from build123d import *

# Parameters (mm, degrees)
SKETCH_1_W         = 25.5
SKETCH_1_H         = 25
EXTRUDE_1_DEPTH    = 4
SKETCH_6_W         = 25.5
SKETCH_6_H         = 7
EXTRUDE_2_DEPTH    = 7
HOLE_WIZARD_M3_1_D = 2.5
HOLE_WIZARD_M4_3_D = 3.3
FILLET_1_R         = 1


with BuildPart() as part:
    # 草图1 → 凸台-拉伸1 (new body)
    with BuildSketch(Plane(origin=(0, 0, 0), x_dir=(1, 0, 0), z_dir=(0, 1, 0))):
        Rectangle(SKETCH_1_W, SKETCH_1_H)
    extrude(amount=EXTRUDE_1_DEPTH)

    # 草图6 → 凸台-拉伸2 (add)
    with BuildSketch(Plane(origin=(0, 4, 0), x_dir=(1, 0, 0), z_dir=(0, 1, 0))):
        with Locations((0, 9)):
            Rectangle(SKETCH_6_W, SKETCH_6_H)
        with Locations((0, -9)):
            Rectangle(SKETCH_6_W, SKETCH_6_H)
    extrude(amount=EXTRUDE_2_DEPTH)

    # M3 螺纹孔1 (through all)
    with Locations(Plane(origin=(6.35, 0, 0), x_dir=(0, 0, -1), z_dir=(0, -1, 0))):
        with Locations((0, 0), (0, -12.7)):
            Hole(HOLE_WIZARD_M3_1_D / 2)

    # M4 螺纹孔3 (through all)
    with Locations(Plane(origin=(7.5, 0, 8.5), x_dir=(0, 0, -1), z_dir=(0, -1, 0))):
        with Locations((0, 0), (0, -15), (17, -15), (17, 0)):
            Hole(HOLE_WIZARD_M4_3_D / 2)

    # 圆角1
    fillet_1_edges = [part.edges().sort_by_distance(p)[0] for p in [
        (0, 4, -5.5),
        (0, 11, -12.5),
        (0, 4, 5.5),
        (0, 11, 12.5),
        (0, 0, 12.5),
        (0, 0, -12.5),
    ]]
    fillet(fillet_1_edges, radius=FILLET_1_R)


solid = part.part
Geometry: final body of the model. Coordinates: model frame, mm. A direction names the side the tool comes from. Coordinates: 2 decimals unless noted, no trailing zeros. Order: outer loops, then holes, each group sorted by start corner. A loop starts at its lowest first (then second) coordinate and runs counter-clockwise, first axis right, second up. Notation, with made-up numbers: M -38.75,70.5 L -10.75,70.5 A32 ccw -10.75,98.5 Z; hole C 75.25,-22 d11. An arc over 180 degrees is marked long. One line per question, with ' | ' between items. Start each with the question number.
Item 1: Ray query, probe 1 along X at (y, z) = (6.75, -8.5); probe 2 along X at (y, z) = (2.55, 0); probe 3 along Z at (x, y) = (-4.75, 7.5). Return the intervals inside material, ascending. Write a range as [from, to].
Item 2: Cut plane C-C, the plane y = 3.5. Return the cut outline in (x, z), then the cut area to 3 significant figures.
Item 3: Cut plane B-B, the plane z = 8.5. Return the cut outline in (x, y), then the cut area to 3 significant figures.
Item 4: Cut plane D-D, the plane x = 6.35. Return the cut outline in (y, z).
Item 5: Draft query along Z for faces 1 (the cylindrical face through (0.178, 10.699, 12.215)), 2 (the flat face through (0, 11, 8)), 3 (the cylindrical face through (8.615, 5.577, 7.284)). Return one class per face: released by +Z, released by -Z, zero draft, split by the parting line, or undercut.
Item 6: Set-up query: faces 4 (the flat face through (12.75, 3, 0)), 5 (the flat face through (0, 8, 5.5)). Return all of +Z, -Z, +X, -X, +Y, -Y with unobstructed straight access to the full face (end or side cutting, diameter ignored); none if empty.
Item 7: Pin query (flat end, axial travel): pin 1 Ø5.5 at (x, z) = (-7.5, 8.5) entering from -Y; pin 2 Ø4 at (x, z) = (-6.35, 0) entering from +Y; pin 3 Ø2 at (x, z) = (6.35, 0) entering from +Y (3 decimals). Return the tip coordinate at first contact, or that it passes through.
Item 8: Cut plane A-A, the plane y = 7.5. Return the cut outline in (x, z).
A:
1) probe 1: x = [-12.75, -9.15], [-5.85, 5.85], [9.15, 12.75] | probe 2: x = [-12.75, -7.6], [-5.1, 5.1], [7.6, 12.75] | probe 3: z = [-12.5, -5.5], [5.5, 12.5]
2) outline: M -12.75,-12.5 L 12.75,-12.5 L 12.75,12.5 L -12.75,12.5 Z; hole C -7.5,-8.5 d3.3; hole C -7.5,8.5 d3.3; hole C -6.35,0 d2.5; hole C 6.35,0 d2.5; hole C 7.5,-8.5 d3.3; hole C 7.5,8.5 d3.3 | area: 593 mm2
3) outline: M -12.75,0 L -9.15,0 L -9.15,11 L -12.75,11 Z; M -5.85,0 L 5.85,0 L 5.85,11 L -5.85,11 Z; M 9.15,0 L 12.75,0 L 12.75,11 L 9.15,11 Z | area: 208 mm2
4) outline: M 0,-11.5 A1 ccw 1,-12.5 L 10,-12.5 A1 ccw 11,-11.5 L 11,-9.68 L 0,-9.68 Z; M 0,-7.32 L 11,-7.32 L 11,-5.5 L 5,-5.5 A1 cw 4,-4.5 L 4,-1.25 L 0,-1.25 Z; M 0,1.25 L 4,1.25 L 4,4.5 A1 cw 5,5.5 L 11,5.5 L 11,7.32 L 0,7.32 Z; M 0,9.68 L 11,9.68 L 11,11.5 A1 ccw 10,12.5 L 1,12.5 A1 ccw 0,11.5 Z
5) face 1: released by +Z | face 2: zero draft | face 3: undercut
6) face 4: +Z, -Z, +X, +Y, -Y | face 5: +X, -X, +Y
7) pin 1: stops at y = 0 | pin 2: stops at y = 4 | pin 3: passes through
8) outline: M -12.75,-12.5 L 12.75,-12.5 L 12.75,-5.5 L -12.75,-5.5 Z; M -12.75,5.5 L 12.75,5.5 L 12.75,12.5 L -12.75,12.5 Z; hole C -7.5,-8.5 d3.3; hole C -7.5,8.5 d3.3; hole C 7.5,-8.5 d3.3; hole C 7.5,8.5 d3.3
